Check sheet for the drawn part. Datum: minimum x, y, z corner. Units: mm. Round coordinates to 2 decimals unless told otherwise and drop trailing zeros. Write each loop counter-clockwise with the first axis right and the second up, starting at its lowest first coordinate (ties: lowest second). Pieces come first, ordered by that corner, then holes. Notation, with made-up numbers: M -19.5,70 L 10.5,70 A22 cw 10.5,92 Z; hole C 70,88 d6. An arc over 180 degrees is marked long. Use a Markdown table: item, result.
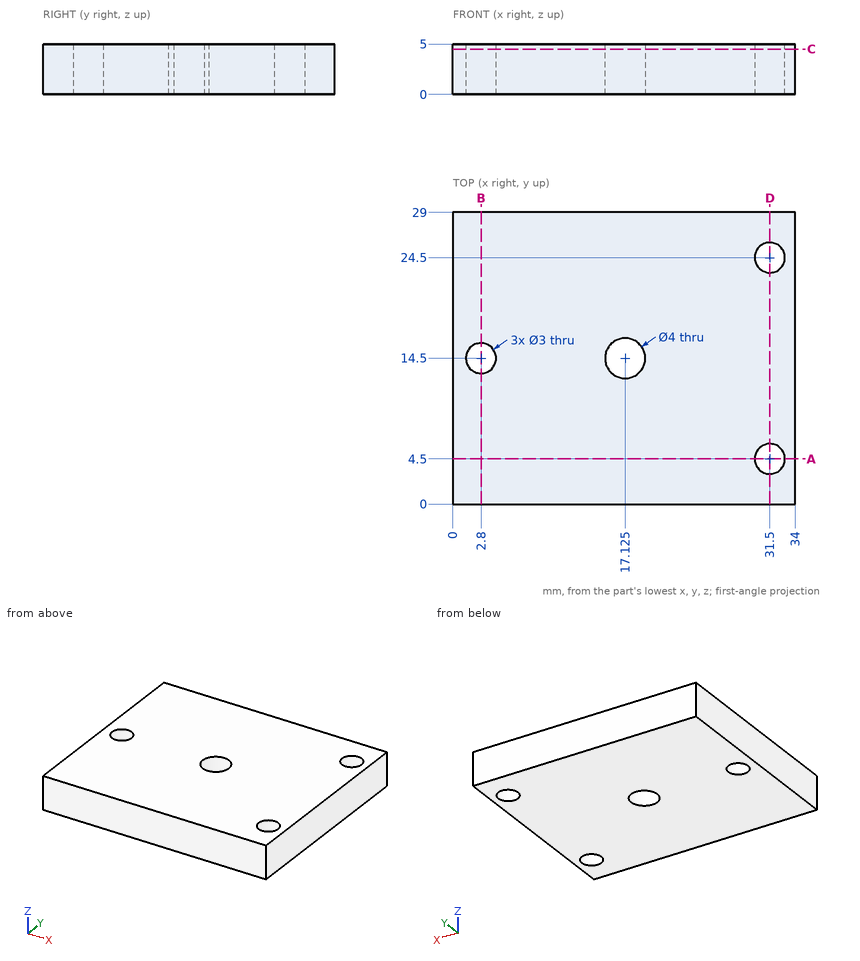
Item 1: Go/stop test with a flat-tipped pin: pin 1 (2.5 mm diameter, centred on x = 17.125, y = 14.5, fed in from +Z). Record where the tip stops, or that it passes through.
Outcome:
| item | result |
|---|---|
| pin 1 | passes through |
Item 2: Cross-section at C-C, the plane z = 4.5. Record the cut outline in (x, y) (3 decimals), and give its area (3 significant figures).
Outcome:
| item | result |
|---|---|
| outline | M 0,0 L 34,0 L 34,29 L 0,29 Z; hole C 2.8,14.5 d3; hole C 17.125,14.5 d4; hole C 31.5,4.5 d3; hole C 31.5,24.5 d3 |
| area | 952 mm2 |
Item 3: Material ranges on line 1 along Y through (x, z) = (31.5, 1.6); line 2 along Y through (x, z) = (2.8, 1.25); line 3 along X through (y, z) = (25, 2), recorded low to high. Write a range as from..to.
Outcome:
| item | result |
|---|---|
| line 1 | y = 0..3, 6..23, 26..29 |
| line 2 | y = 0..13, 16..29 |
| line 3 | x = 0..30.09, 32.91..34 |
Item 4: Cross-section at A-A, the plane y = 4.5. Record the cut outline in (x, z), and give its area (3 significant figures).
Outcome:
| item | result |
|---|---|
| outline | M 0,0 L 30,0 L 30,5 L 0,5 Z; M 33,0 L 34,0 L 34,5 L 33,5 Z |
| area | 155 mm2 |
Item 5: Cross-section at B-B, the plane x = 2.8. Record the cut outline in (y, z), and give its area (3 significant figures).
Outcome:
| item | result |
|---|---|
| outline | M 0,0 L 13,0 L 13,5 L 0,5 Z; M 16,0 L 29,0 L 29,5 L 16,5 Z |
| area | 130 mm2 |
Item 6: Cross-section at D-D, the plane x = 31.5. Record the cut outline in (y, z).
Outcome:
| item | result |
|---|---|
| outline | M 0,0 L 3,0 L 3,5 L 0,5 Z; M 6,0 L 23,0 L 23,5 L 6,5 Z; M 26,0 L 29,0 L 29,5 L 26,5 Z |
